Source: CAD feature listing. Evaluate the final solid. Frame: model axes, mm. Round coordinates to 2 decimals unless told otherwise and drop trailing zeros. Write each loop counter-clockwise with the first axis right and the second up, starting at its lowest first coordinate (ties: lowest second). Pieces come first, ordered by that corner, then holes.
from build123d import *

# Parameters (mm, degrees)
IZIM1_W               = 300
IZIM1_H               = 150
TABAN_FLAN_1_DEPTH    = 10
IZIM6_R               = 28
KES_EKSTR_ZYON1_DEPTH = 10
IZIM7_R               = 7.5
KES_EKSTR_ZYON2_DEPTH = 15
IZIM8_W               = 17.5
IZIM8_H               = 43
IZIM8_W_2             = 195
SEKME1_DEPTH          = 10


# Sheet-metal steps are written as plain solids
with BuildPart() as part:
    # Çizim1 → Taban-Flanş1 (new body)
    with BuildSketch(Plane.XY):
        Rectangle(IZIM1_W, IZIM1_H)
    extrude(amount=-TABAN_FLAN_1_DEPTH)

    # Çizim6 → Kes-Ekstrüzyon1 (cut)
    with BuildSketch(Plane(origin=(0, 0, -10), x_dir=(-1, 0, 0), z_dir=(0, 0, -1))):
        with Locations((-55, -5)):
            Circle(IZIM6_R)
        with Locations((55, -5)):
            Circle(IZIM6_R)
    extrude(amount=-KES_EKSTR_ZYON1_DEPTH, mode=Mode.SUBTRACT)

    # Çizim7 → Kes-Ekstrüzyon2 (cut)
    with BuildSketch(Plane(origin=(0, 0, -10), x_dir=(-1, 0, 0), z_dir=(0, 0, -1))):
        with Locations((-137, 40)):
            Circle(IZIM7_R)
        with Locations((-137, -35)):
            Circle(IZIM7_R)
    kes_ekstr_zyon2 = extrude(amount=-KES_EKSTR_ZYON2_DEPTH, mode=Mode.SUBTRACT)

    # Aynalama1: Kes-Ekstrüzyon2 across plane
    add(kes_ekstr_zyon2.mirror(Plane(origin=(0, 0, 0), x_dir=(0, 0, 1), z_dir=(1, 0, 0))), mode=Mode.SUBTRACT)

    # Çizim8 → Sekme1 (add)
    with BuildSketch(Plane(origin=(0, 0, -10), x_dir=(-1, 0, 0), z_dir=(0, 0, -1))):
        with Locations((-141.25, -96.5)):
            Rectangle(IZIM8_W, IZIM8_H)
        with Locations((0, -96.5)):
            Rectangle(IZIM8_W_2, IZIM8_H)
        with Locations((141.25, -96.5)):
            Rectangle(IZIM8_W, IZIM8_H)
    extrude(amount=-SEKME1_DEPTH)


solid = part.part
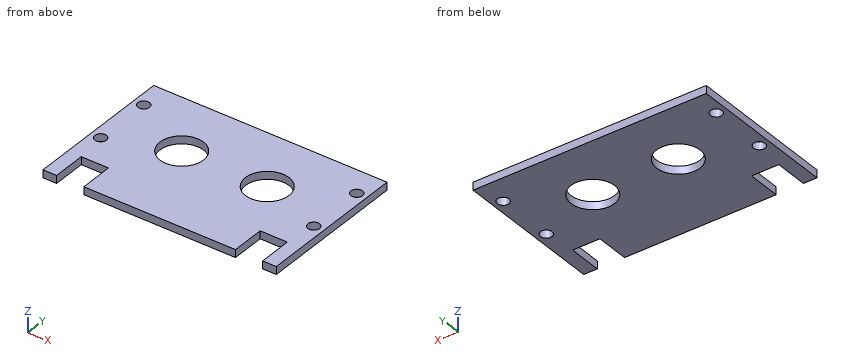
1) Contact query for a flat-ended pin moving along its axis: P1, Ø3, axis at x = -114, z = -5.5, coming from the -Y side. Output: stop coordinate, or through.
Taken from the geometry:
P1: stops at y = -75
2) Material intervals for line 1 (Y direction, x = 137, z = -6); line 2 (X direction, y = -83.5, z = -5.5); line 3 (X direction, y = 38, z = -8.25), sorted ascending.
Taken from the geometry:
line 1: y = -118 to -42.5, -27.5 to 32.5, 47.5 to 75
line 2: x = -150 to -132.5, -97.5 to 97.5, 132.5 to 150
line 3: x = -150 to -144.23, -129.77 to 129.77, 144.23 to 150
3) Section query D-D on y = 40. Return the cut outline in (x, z), then the cut area to 3 significant figures.
Taken from the geometry:
outline: (-150, -10) - (-144.5, -10) - (-144.5, 0) - (-150, 0) - close; (-129.5, -10) - (129.5, -10) - (129.5, 0) - (-129.5, 0) - close; (144.5, -10) - (150, -10) - (150, 0) - (144.5, 0) - close
area: 2,700 mm2
4) Section query A-A on x = 137. Return the cut outline in (y, z).
Taken from the geometry:
outline: (-118, -10) - (-42.5, -10) - (-42.5, 0) - (-118, 0) - close; (-27.5, -10) - (32.5, -10) - (32.5, 0) - (-27.5, 0) - close; (47.5, -10) - (75, -10) - (75, 0) - (47.5, 0) - close
5) Section query C-C on x = 55. Return the cut outline in (y, z).
Taken from the geometry:
outline: (-118, -10) - (-33, -10) - (-33, 0) - (-118, 0) - close; (23, -10) - (75, -10) - (75, 0) - (23, 0) - close
6) Section query B-B on z = -6.75. Return the cut outline in (x, y).
Taken from the geometry:
outline: (-150, -118) - (-132.5, -118) - (-132.5, -75) - (-97.5, -75) - (-97.5, -118) - (97.5, -118) - (97.5, -75) - (132.5, -75) - (132.5, -118) - (150, -118) - (150, 75) - (-150, 75) - close; hole circle Ø15 at (-137, -35); hole circle Ø15 at (-137, 40); hole circle Ø56 at (-55, -5); hole circle Ø56 at (55, -5); hole circle Ø15 at (137, -35); hole circle Ø15 at (137, 40)
